```python
from build123d import *

# Parameters (mm, degrees)
F0_W     = 19.05
F0_H     = 19.05
F1_DEPTH = 9.525


with BuildPart() as f1:
    # F0 (on Front) → F1 (new body, symmetric)
    with BuildSketch(Plane.XZ):
        Polygon((0, 19.05), (-19.05, 19.05), (-19.05, 0.013117), (-19.05, -19.036883), (-19.05, -19.05), (0, -19.05), (19.05, -19.05), (19.05, 19.05), align=None)
        with Locations((9.525, 28.575)):
            Rectangle(F0_W, F0_H)
        with Locations((-28.575, -9.511883)):
            Rectangle(F0_W, F0_H)
    extrude(amount=F1_DEPTH, both=True)


solid = f1.part
```
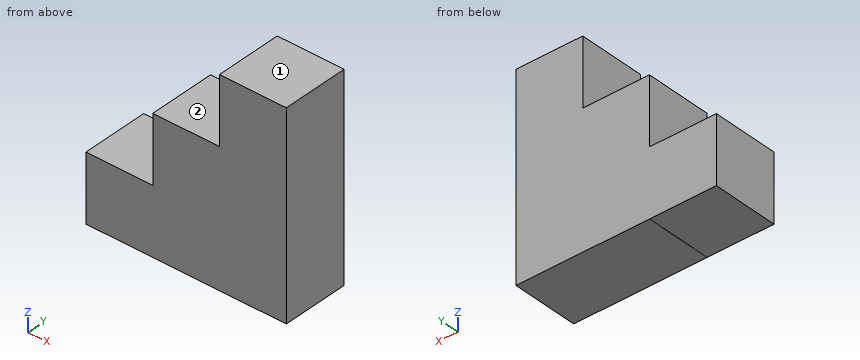
Model file for the job. Use its own axes, mm. Face numbers are marked on the shaded views. A direction names the side the tool comes from. Give positions to 0.01 mm unless a question says otherwise; leave off trailing zeros. Loops run counter-clockwise (first coordinate to the right, second up) from the corner with the lowest first, then second, coordinate; pieces in that order, holes last. Notation, with made-up numbers: (13.5, 83.5) -> (17.5, 83.5) arc R18 ccw to (17.5, 92.5) -> close; hole circle Ø8 at (-26.75, -10). An arc over 180 degrees is marked (long way). Write each question's results on one line, items separated by ' | '.
(1) Probe line 1 along X through (y, z) = (-1.75, 1); line 2 along Z through (x, y) = (-35, 3.25). List the from-to ranges inside material, lowest first.
Geometry results:
line 1: x = -19.05 to 19.05 | line 2: z = -19.04 to 0.01
(2) Flat gauge pins, fed straight in: pin 1 Ø9.5 at (x, y) = (-5, 3.5) entering from +Z; pin 2 Ø9.5 at (y, z) = (0, 24.5) entering from -X; pin 3 Ø5 at (x, y) = (-27.5, 4.5) entering from -Z. Where does each tip first touch, or does it go through?
Geometry results:
pin 1: stops at z = 19.05 | pin 2: stops at x = 0 | pin 3: stops at z = -19.04
(3) Tool access for the marked faces 1 and 2: list every direction of +Z, -Z, +X, -X, +Y, -Y with a clear straight run to the whole face (end or side of a thin tool).
Geometry results:
face 1: +Z, +X, -X, +Y, -Y | face 2: +Z, -X, +Y, -Y
(4) Cut at B-B on z = 5. List the corners of the cut face in (x, y) (3 decimals), and give its area (3 significant figures).
Geometry results:
outline: (-19.05, -9.525) -> (19.05, -9.525) -> (19.05, 9.525) -> (-19.05, 9.525) -> close | area: 726 mm²
(5) Cut at C-C on z = 20. List the corners of the cut face in (x, y) (3 decimals), and give its area (3 significant figures).
Geometry results:
outline: (0, -9.525) -> (19.05, -9.525) -> (19.05, 9.525) -> (0, 9.525) -> close | area: 363 mm²
